Part print with two shaded views. Sizes in mm from the minimum x, y, z corner. A direction names the side the tool comes from. Coordinates: 2 decimals unless noted, no trailing zeros. Write each loop counter-clockwise with the first axis right and the second up, starting at its lowest first coordinate (ties: lowest second). Pieces come first, ordered by that corner, then holes. Notation, with made-up numbers: (-30, 37.25) - (-13, 37.25) arc R5 ccw to (-13, 46.25) - close; hole circle Ø6 at (58, 78). An arc over 180 degrees is marked (long way). Answer in a Markdown table with one row per item. Add a question column.
Q1. 3-axis set-ups, long thin cutter, end or side, ignore diameter. For the marked faces 1 and 2: which of +Z, -Z, +X, -X, +Y, -Y reach the whole face in a straight line?
Q2. Band-saw the part on C-C (z = 4). List the corners of the cut face in (x, y).
Q3. Band-saw the part on D-D (z = 8). List the corners of the cut face in (x, y), and give its area (3 significant figures).
Q4. Drill centre lines: line 1 along Z through (x, y) = (9.5, 3.75); line 2 along X through (y, z) = (9.75, 2.5); line 3 along Z through (x, y) = (0.75, 4.5). Where is each one in solid material? Low to high. Write a range as from..to.
Q5. Pin check, flat tips, straight feed: pin 1 (1 mm diameter, centred on x = 11, z = 5, fed in from +Y); pin 2 (1.5 mm diameter, centred on y = 3.5, z = 6.5, fed in from +X); pin 3 (5 mm diameter, centred on y = 10.5, z = 1.5, fed in from -X). Stop position of each tip, or through.
Q6. Band-saw the part on A-A (x = 7). List the corners of the cut face in (y, z).
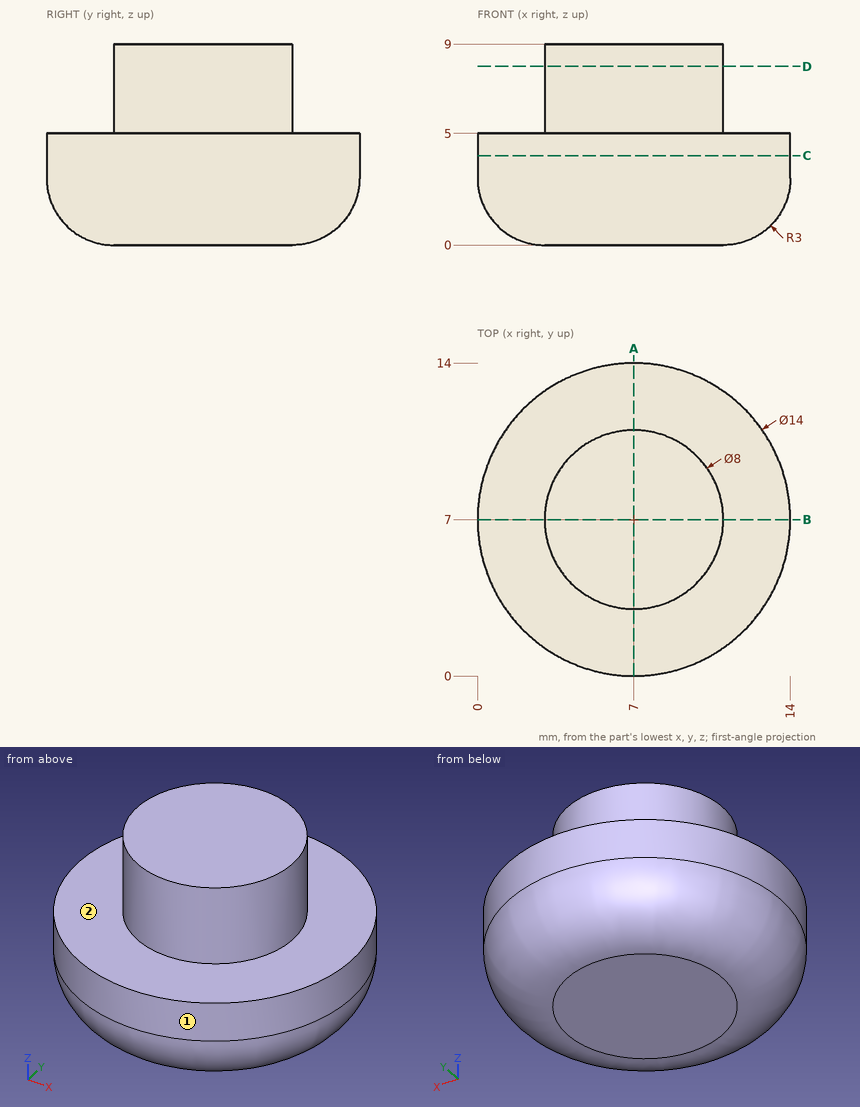
Checked values:
| question | item | result |
|---|---|---|
| 1 | face 1 | +Z, -Z |
| 1 | face 2 | +Z |
| 2 | outline | circle Ø14 at (7, 7) |
| 3 | outline | circle Ø8 at (7, 7) |
| 3 | area | 50.3 mm² |
| 4 | line 1 | z = 0..5 |
| 4 | line 2 | x = 0.61..13.39 |
| 4 | line 3 | z = 1.76..5 |
| 5 | pin 1 | stops at y = 13.06 |
| 5 | pin 2 | stops at x = 9.9 |
| 5 | pin 3 | stops at x = 0.14 |
| 6 | outline | (0, 3) arc R3 ccw to (3, 0) - (11, 0) arc R3 ccw to (14, 3) - (14, 5) - (11, 5) - (11, 9) - (3, 9) - (3, 5) - (0, 5) - close |
